Verification items for the finished model (mm, model axes). A direction names the side the tool comes from. Round coordinates to 2 decimals unless told otherwise and drop trailing zeros. Loops run counter-clockwise (first coordinate to the right, second up) from the corner with the lowest first, then second, coordinate; pieces in that order, holes last. Notation, with made-up numbers: (54, 65.5) -> (59, 65.5) arc R15 cw to (59, 87.5) -> close; hole circle Ø10 at (17.5, -15). An arc over 180 degrees is marked (long way). Write item = value, one per line.
```python
from build123d import *

# Parameters (mm, degrees)
SKETCH1_W           = 40
SKETCH1_H           = 30
SKETCH1_R           = 1.5
BOSS_EXTRUDE1_DEPTH = 15
SKETCH2_W           = 30
SKETCH2_H           = 30
CUT_EXTRUDE1_DEPTH  = 12
SKETCH3_W           = 10
SKETCH3_H           = 10
CUT_EXTRUDE2_DEPTH  = 12
CUT_EXTRUDE3_DEPTH  = 12


with BuildPart() as part:
    # Sketch1 → Boss-Extrude1 (new body)
    with BuildSketch(Plane(origin=(0, 0, 0), x_dir=(1, 0, 0), z_dir=(0, 1, 0))):
        with Locations((-39.556208855, 16.822571299)):
            Rectangle(SKETCH1_W, SKETCH1_H)
        with Locations(Location((-24.556208855, 26.822571299, 0), (0, 0, 270))):
            Circle(SKETCH1_R, mode=Mode.SUBTRACT)
        with Locations(Location((-24.556208855, 6.822571299, 0), (0, 0, 270))):
            Circle(SKETCH1_R, mode=Mode.SUBTRACT)
    extrude(amount=BOSS_EXTRUDE1_DEPTH)

    # Sketch2 → Cut-Extrude1 (cut)
    with BuildSketch(Plane(origin=(0, 15, 0), x_dir=(1, 0, 0), z_dir=(0, 1, 0))):
        with Locations((-44.556208855, 16.822571299)):
            Rectangle(SKETCH2_W, SKETCH2_H)
    extrude(amount=-CUT_EXTRUDE1_DEPTH, mode=Mode.SUBTRACT)

    # Sketch3 → Cut-Extrude2 (cut)
    with BuildSketch(Plane(origin=(0, 15, 0), x_dir=(1, 0, 0), z_dir=(0, 1, 0))):
        with Locations((-24.556208855, 16.822571299)):
            Rectangle(SKETCH3_W, SKETCH3_H)
    extrude(amount=-CUT_EXTRUDE2_DEPTH, mode=Mode.SUBTRACT)

    # Sketch4 → Cut-Extrude3 (cut)
    with BuildSketch(Plane(origin=(0, 15, 0), x_dir=(1, 0, 0), z_dir=(0, 1, 0))):
        Polygon((-23.899354605, 21.822571299), (-19.556208855, 26.165717049), (-19.556208855, 21.822571299), align=None)
        Polygon((-23.899354605, 11.822571299), (-19.556208855, 7.479425548), (-19.556208855, 11.822571299), align=None)
    extrude(amount=-CUT_EXTRUDE3_DEPTH, mode=Mode.SUBTRACT)


solid = part.part
```
(1) Sectioned sample at C-C, the plane z = -19.5. Record the cut outline in (x, y), and give its area (3 significant figures).
Filled sheet:
outline = (-59.56, 0) -> (-19.56, 0) -> (-19.56, 3) -> (-59.56, 3) -> close
area = 120 mm2
(2) Material ranges on probe 1 along X at (y, z) = (10.75, -27); probe 2 along Z at (x, y) = (-29, 12.5); probe 3 along X at (y, z) = (8.5, -6.75), recorded low to high. Write a range as from..to.
Filled sheet:
probe_1 = -29.56..-26.05, -23.07..-19.56
probe_2 = -31.82..-21.82, -11.82..-1.82
probe_3 = -29.56..-26.05, -23.06..-19.56
(3) Set-up check for faces 4 (the face through (-21.76, 9.08, -23.96)), 5 (the face through (-31, 2, -31.823)), 6 (the face through (-29.556, 9, -27)), 7 (the face through (-27, 9, -21.823)): record each of +Z, -Z, +X, -X, +Y, -Y from which the full face is reachable in a straight line by a thin tool's end or side.
Filled sheet:
face_4 = +X, +Y
face_5 = -Z, +X, -X, +Y, -Y
face_6 = +Z, -Z, -X, +Y
face_7 = +X, -X, +Y
(4) Go/stop test with flat-tipped pins: pin 1 Ø5 at (y, z) = (7, -7) entering from -X; pin 2 Ø5 at (x, y) = (-32, 3.5) entering from -Z; pin 3 Ø4 at (x, z) = (-55.5, -15.5) entering from +Y. Record where each tip stops, or that it passes through.
Filled sheet:
pin_1 = -29.56
pin_2 = -31.82
pin_3 = 3
(5) Draft check along Z on faces 1 (the face through (-19.556, 2, -17)), 2 (the face through (-31, 2, -1.823)), 3 (the face through (-27, 9, -11.823)). Enter one of: released by +Z, released by -Z, zero draft, split by the parting line, or undercut.
Filled sheet:
face_1 = zero draft
face_2 = released by +Z
face_3 = undercut
(6) Sectioned sample at B-B, the plane x = -53. Record the cut outline in (y, z), and give its area (3 significant figures).
Filled sheet:
outline = (0, -31.82) -> (3, -31.82) -> (3, -1.82) -> (0, -1.82) -> close
area = 90.0 mm2
(7) Sectioned sample at A-A, the plane y = 14.25. Record the cut outline in (x, z).
Filled sheet:
outline = (-29.56, -31.82) -> (-19.56, -31.82) -> (-19.56, -26.17) -> (-23.9, -21.82) -> (-29.56, -21.82) -> close; (-29.56, -11.82) -> (-23.9, -11.82) -> (-19.56, -7.48) -> (-19.56, -1.82) -> (-29.56, -1.82) -> close; hole circle Ø3 at (-24.56, -26.82); hole circle Ø3 at (-24.56, -6.82)
